Design review of the part built by this model. Coordinates are the model's own, in mm. A direction names the side the tool comes from. Round coordinates to 2 decimals unless told otherwise and drop trailing zeros. Order: outer loops, then holes, each group sorted by start corner. A loop starts at its lowest first (then second) coordinate and runs counter-clockwise, first axis right, second up. Notation, with made-up numbers: (70, 23.5) - (81, 23.5) arc R19 cw to (81, 42.5) - close; hole circle Ø2 at (51, 6.5). An arc over 180 degrees is marked (long way). Write item = value, one per line.
from build123d import *

# Parameters (mm, degrees)
SKETCH1_W                               = 20
SKETCH1_H                               = 8
EXTRUDE1_DEPTH                          = 8
SKETCH2_W                               = 14
SKETCH2_H                               = 8
EXTRUDE2_DEPTH                          = 3.5
CBORE_FOR_M5_HEX_HEAD_BOLT1_D           = 3
CBORE_FOR_M5_HEX_HEAD_BOLT1_CBORE_D     = 6.5
CBORE_FOR_M5_HEX_HEAD_BOLT1_CBORE_DEPTH = 3


with BuildPart() as part:
    # Sketch1 → Extrude1 (new body)
    with BuildSketch(Plane.XY):
        Rectangle(SKETCH1_W, SKETCH1_H)
    extrude(amount=-EXTRUDE1_DEPTH)

    # Sketch2 → Extrude2 (cut)
    with BuildSketch(Plane(origin=(0, 0, -8), x_dir=(-1, 0, 0), z_dir=(0, 0, -1))):
        Rectangle(SKETCH2_W, SKETCH2_H)
    extrude(amount=-EXTRUDE2_DEPTH, mode=Mode.SUBTRACT)

    # CBORE for M5 Hex Head Bolt1 (through all)
    with Locations(Plane.XY):
        with Locations((0, 0)):
            CounterBoreHole(CBORE_FOR_M5_HEX_HEAD_BOLT1_D / 2, CBORE_FOR_M5_HEX_HEAD_BOLT1_CBORE_D / 2, CBORE_FOR_M5_HEX_HEAD_BOLT1_CBORE_DEPTH)


solid = part.part
Item 1: Take a section at B-B, the plane x = 0. State the section outline as (y, z) points, and give its area (3 significant figures).
Data:
outline = (-4, -4.5) - (-1.5, -4.5) - (-1.5, -3) - (-3.25, -3) - (-3.25, 0) - (-4, 0) - close; (1.5, -4.5) - (4, -4.5) - (4, 0) - (3.25, 0) - (3.25, -3) - (1.5, -3) - close
area = 12.0 mm2
Item 2: Take a section at D-D, the plane z = -0.5. State the section outline as (x, y) points, and give its area (3 significant figures).
Data:
outline = (-10, -4) - (10, -4) - (10, 4) - (-10, 4) - close; hole circle Ø6.5 at (0, 0)
area = 127 mm2
Item 3: For faces 4 (the face through (8, 0, -8)), 5 (the face through (2, 0, -4.5)), 6 (the face through (-2.579, -1.978, -1.479)), list the 3-axis set-ups (+Z, -Z, +X, -X, +Y, -Y) from which the entire face can be reached by the end or side of a thin tool; tool diameter is ignored.
Data:
face_4 = -Z, +X, -X, +Y, -Y
face_5 = -Z, +Y, -Y
face_6 = +Z
Item 4: The part is to be moulded in two halves that separate along X. For faces 1 (the face through (0.7, 1.5, -3)), 2 (the face through (0, -4, -3)), 3 (the face through (10, 0, -4)), say which applies: +X half, -X half, draft (parallel to the pull), parting line (faces both ways), or undercut.
Data:
face_1 = undercut
face_2 = draft
face_3 = +X half
Item 5: Take a section at A-A, the plane y = 0. State the section outline as (x, z) points.
Data:
outline = (-10, -8) - (-7, -8) - (-7, -4.5) - (-1.5, -4.5) - (-1.5, -3) - (-3.25, -3) - (-3.25, 0) - (-10, 0) - close; (1.5, -4.5) - (7, -4.5) - (7, -8) - (10, -8) - (10, 0) - (3.25, 0) - (3.25, -3) - (1.5, -3) - close
Item 6: For line 1 along Y through (x, z) = (0, -3.9); line 2 along Y through (x, z) = (0, -0.7); line 3 along X through (y, z) = (3, -6.5), list the stretches that pass through material, from the lowest coordinate up. Write a range as [from, to].
Data:
line_1 = [-4, -1.5], [1.5, 4]
line_2 = [-4, -3.25], [3.25, 4]
line_3 = [-10, -7], [7, 10]
Item 7: Take a section at C-C, the plane z = -5.25. State the section outline as (x, y) points, and give its area (3 significant figures).
Data:
outline = (-10, -4) - (-7, -4) - (-7, 4) - (-10, 4) - close; (7, -4) - (10, -4) - (10, 4) - (7, 4) - close
area = 48.0 mm2
Item 8: Insertion check: P1, Ø4, axis at x = 0, y = 0, coming from the +Z side; P2, Ø1.5, axis at x = -1, y = 1.5, coming from the -Z side. Each pin has a flat end and moves straight along its axis. Give the tip position at first contact, or say it passes through.
Data:
P1 = -3
P2 = -4.5
